Autodesk Inventor part; units mm, degrees
ref_plane "Plano inicial" through (0, 0, 0) normal (0, 0, 1) x (1, 0, 0)
ref_plane "Plano final" through (0, 0, 550) normal (0, 0, 1) x (1, 0, 0)
ref_plane "Plano de trabalho6" through (-155, 0, 0) normal (0, 0, -1) x (-1, 0, 0)
ref_plane "Plano inicial" through (0, 0, 0) normal (0, 0, 1) x (1, 0, 0)
ref_plane "Plano final" through (0, 0, 550) normal (0, 0, 1) x (1, 0, 0)
sketch "Esboço" plane through (0, 0, 0) normal (0, 0, 1) x (1, 0, 0)
  line L0 (-15, -11) -> (-15, 11)
  line L1 (-11, 15) -> (11, 15)
  line L2 (15, 11) -> (15, -11)
  line L3 (11, -15) -> (-11, -15)
  arc A0 (-15, -11) -> (-11, -15) centre (-11, -11) ccw
  arc A1 (15, 11) -> (11, 15) centre (11, 11) ccw
  arc A2 (-11, 15) -> (-15, 11) centre (-11, 11) ccw
  arc A3 (11, -15) -> (15, -11) centre (11, -11) ccw
  arc A4 (-11, 13) -> (-13, 11) centre (-11, 11) ccw
  line L4 (-11, 13) -> (11, 13)
  arc A5 (13, 11) -> (11, 13) centre (11, 11) ccw
  line L5 (13, 11) -> (13, -11)
  arc A6 (11, -13) -> (13, -11) centre (11, -11) ccw
  line L6 (11, -13) -> (-11, -13)
  arc A7 (-13, -11) -> (-11, -13) centre (-11, -11) ccw
  line L7 (-13, -11) -> (-13, 11)
  line L8 (0, 22.1598) -> (0, -22.1598) construction
  line L9 (-22.1598, 0) -> (22.1598, 0) construction
  dimension "d7" = 4
  dimension "d9" = 30
  dimension "d11" = 30
  dimension "d12" = 2
  dimension "d15" = 15
  dimension "d16" = 15
extrude "Corpo" add sketch "Esboço" along normal up to surface (550 mm away) from surface at 0
sketch "Sketch3" plane through (0, 0, 0) normal (0, 0, 1) x (1, 0, 0)
  line L0 (0, 0) -> (10, 0)
ref_plane "Work Plane3" through (0, 0, 0) normal (0, -1, 0) x (1, 0, 0)
sketch "Sketch4" plane through (0, 0, 0) normal (0, -1, 0) x (1, 0, 0)
  line L0 (-2, 0) -> (12, 0)
  line L1 (-2, 550) -> (12, 550)
  dimension "d18" = 550
ref_plane "Plano de trabalho6" through (-155, 0, 0) normal (0, 0, -1) x (-1, 0, 0)
split "Dividir3" plane through (-155, 0, 0) removes the side toward (0, 0, -1)
ref_plane "Plano de trabalho7" through (-15, 0, 550) normal (0, 0, 1) x (1, 0, 0)
split "Dividir4" plane through (-15, 0, 550) removes the side toward (0, 0, 1)
ref_plane "Plano de trabalho8" through (0, 15, 550) normal (0, -0.7071, 0.7071) x (1, 0, 0)
split "Dividir5" plane through (0, 15, 550) removes the side toward (0, -0.7071, 0.7071)
ref_plane "Plano de trabalho9" through (0, 15, 0) normal (0, -0.7071, -0.7071) x (1, 0, 0)
split "Dividir6" plane through (0, 15, 0) removes the side toward (0, -0.7071, -0.7071)
equation "\"d7\" = G_IR"
equation "\"d9\" = G_W"
equation "\"d11\" = G_H"
equation "\"d12\" = G_T"
equation "\"d15\" = 0.5 * d9"
equation "\"d16\" = 0.5 * d11"
equation "\"d3\" = G_L"
equation "\"G_W\" = 30"
equation "\"G_H\" = 30"
equation "\"G_T\" = 2"
equation "\"G_IR\" = 4"
equation "\"G_L\" = d18"
equation "\"G_OFFSET_START\" = 0"
equation "\"G_OFFSET_END\" = 0"
properties part number "ISO 10799-2 - 30x30x2 - 550" material "Aço, suave"
Model file for the job. Use its own axes, mm. A direction names the side the tool comes from. Give positions to 0.01 mm unless a question says otherwise; leave off trailing zeros. Loops run counter-clockwise (first coordinate to the right, second up) from the corner with the lowest first, then second, coordinate; pieces in that order, holes last. Notation, with made-up numbers: (-26.75, 46.25) -> (17.25, 46.25) arc R12 cw to (17.25, 64.25) -> close; hole circle Ø5 at (50.5, -32). An arc over 180 degrees is marked (long way). Use CSV: the item, a comma, the result in double quotes. Start each with the question number.
1) Flat gauge pins, fed straight in: pin 1 Ø10 at (x, y) = (6, 8.5) entering from -Z; pin 2 Ø10 at (x, y) = (7.5, 2.5) entering from +Z. Where does each tip first touch, or does it go through?
2) Slice it at C-C on z = 65. Give the cut face in (x, y), plus the area to 3 significant figures.
3) Slice it at B-B on x = -4. Give the cut face in (y, z), plus the area to 3 significant figures.
4) Wall check: line 1 (Y direction, x = -10, z = 290.5); line 2 (X direction, y = -12.5, z = 470). Give the ranges that are in metal, low to high.
5) Slice it at A-A on y = -5.75. Give the cut face in (x, z).
6) Mould opens along X. For faces 3 (the flat face through (-14, 0, 535)), 4 (the flat face through (0, 13, 271)), 5 (the flat face through (-15, 0, 271)) say: released by +X, released by -X, zero draft, split by the parting line, or undercut.
7) Tool access for faces 1 (the flat face through (-14, 0, 15)), 2 (the flat face through (0, -13, 272)): list every direction of +Z, -Z, +X, -X, +Y, -Y with a clear straight run to the whole face (end or side of a thin tool).
Computed values:
1,pin 1,"stops at z = 1.5"
1,pin 2,"passes through"
2,outline,"(-15, -11) arc R4 ccw to (-11, -15) -> (11, -15) arc R4 ccw to (15, -11) -> (15, 11) arc R4 ccw to (11, 15) -> (-11, 15) arc R4 ccw to (-15, 11) -> close; hole (-13, -11) arc R2 ccw to (-11, -13) -> (11, -13) arc R2 ccw to (13, -11) -> (13, 11) arc R2 ccw to (11, 13) -> (-11, 13) arc R2 ccw to (-13, 11) -> close"
2,area,"214 mm^2"
3,outline,"(-15, 30) -> (-13, 28) -> (-13, 522) -> (-15, 520) -> close; (13, 2) -> (15, 0) -> (15, 550) -> (13, 548) -> close"
3,area,"2,080 mm^2"
4,line 1,"y = -15 to -13, 13 to 15"
4,line 2,"x = -14.71 to -12.32, 12.32 to 14.71"
5,outline,"(-15, 20.75) -> (-13, 20.75) -> (-13, 529.25) -> (-15, 529.25) -> close; (13, 20.75) -> (15, 20.75) -> (15, 529.25) -> (13, 529.25) -> close"
6,face 3,"zero draft"
6,face 4,"undercut"
6,face 5,"released by -X"
7,face 1,"-Z, +X, -X, -Y"
7,face 2,"+Z, -Z"
